Autodesk Inventor part; units mm, degrees
ref_plane "Work Plane1" through (16.75, 3.375, -6.9) normal (1, 0, 0) x (0, 1, 0)
ref_plane "YZ Plane" through (0, 0, 0) normal (1, 0, 0) x (0, 1, 0)
ref_plane "XZ Plane" through (0, 0, 0) normal (0, 1, 0) x (-1, 0, 0)
sketch "Sketch1" plane through (0, 0, 0) normal (0, 1, 0) x (-1, 0, 0)
  line L0 (11.5, 34.5) -> (-11.5, 34.5)
  line L1 (-11.5, 34.5) -> (-11.5, -34.5)
  line L2 (-11.5, -34.5) -> (11.5, -34.5)
  line L3 (11.5, -34.5) -> (11.5, 34.5)
  line L4 (11.5, 34.5) -> (-11.5, -34.5) construction
  line L5 (-11.5, 34.5) -> (11.5, -34.5) construction
  point P0 (0, 0)
  dimension "d0" = 23
  dimension "d1" = 69
extrude "Extrusion1" add sketch "Sketch1" along normal blind 16
sketch "Sketch3" plane through (11.5, 0, 34.5) normal (1, 0, 0) x (0, 0, -1)
  line L0 (0, 0) -> (69, 0)
  line L1 (69, 0) -> (69, 16)
  line L2 (0, 16) -> (69, 16)
  line L3 (0, 0) -> (0, 16)
  line L4 (41.4, 13.119) -> (36.4, 13.119)
  line L5 (36.4, 13.119) -> (36.4, 11.6808)
  line L6 (36.4, 11.6668) -> (36.4, 3.375)
  line L7 (41.4, 2.875) -> (36.4, 2.875)
  line L8 (36.4, 3.375) -> (36.4, 2.875)
  line L9 (0, 0) -> (0, 16)
  line L10 (36.4, 13.119) -> (0, 13.119)
  line L11 (0, 13.119) -> (0, 2.875)
  line L12 (0, 2.875) -> (36.4, 2.875)
  line L13 (36.4, 2.875) -> (36.4, 13.119)
  point P0 (34.5, 0)
ref_plane "Work Plane1" through (16.75, 3.375, -6.9) normal (1, 0, 0) x (0, 1, 0)
extrude "Extrusion2" add sketch "Sketch3" along normal up to surface (5.25 mm away) contours L3 L10 L5 L13 L6 L8 L12
properties part number "bigLipo"
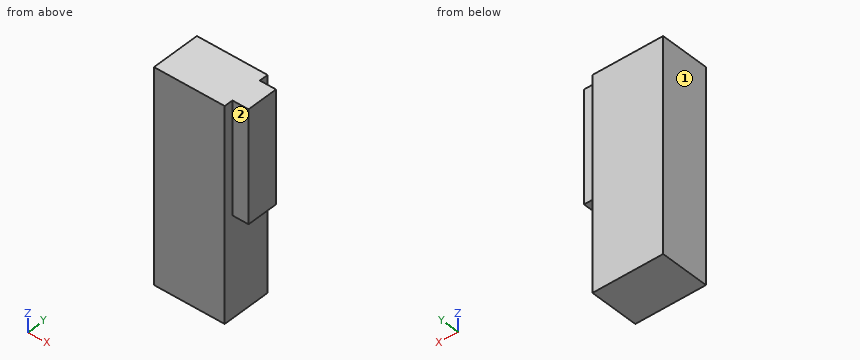
Part model, mm, in its own coordinate system. Face numbers are marked on the shaded views. A direction names the side the tool comes from. Round coordinates to 2 decimals unless told otherwise and drop trailing zeros. Order: outer loops, then holes, each group sorted by start corner. A loop starts at its lowest first (then second) coordinate and runs counter-clockwise, first axis right, second up. Notation, with made-up numbers: M 33,12.5 L 90,12.5 A13 cw 90,31.5 Z; hole C -27.5,70.5 d3. An arc over 180 degrees is marked long. Answer in a Markdown table with one row per item. Add a question column.
Q1. Wall check: L1, parallel to X at y = 10.5, z = -25. Give the ranges that are in metal, low to high. Write a range as from..to.
Q2. Cut at B-B on z = 25.5. Give the cut face in (x, y) (3 decimals), and give its area (3 significant figures).
Q3. Cut at A-A on y = 3.75. Give the cut face in (x, z), and give its area (3 significant figures).
Q4. 3-axis set-ups, long thin cutter, end or side, ignore diameter. For the marked faces 1 and 2: which of +Z, -Z, +X, -X, +Y, -Y reach the whole face in a straight line?
Q5. Cut at D-D on z = -25. Give the cut face in (x, y).
Q6. Cut at C-C on x = 13.5. Give the cut face in (y, z) (3 decimals).
Q7. Pin check, flat tips, straight feed: pin 1 (10 mm diameter, centred on x = 12, z = -15, fed in from +Y); pin 2 (1.6 mm diameter, centred on x = 14.5, z = 17, fed in from +Y). Stop position of each tip, or through.
Established:
| question | item | result |
|---|---|---|
| 1 | L1 | x = -11.5..11.5 |
| 2 | outline | M -11.5,0 L 11.5,0 L 11.5,2.875 L 16.75,2.875 L 16.75,13.119 L 11.5,13.119 L 11.5,16 L -11.5,16 Z |
| 2 | area | 422 mm2 |
| 3 | outline | M -11.5,-34.5 L 11.5,-34.5 L 11.5,-1.9 L 16.75,-1.9 L 16.75,34.5 L -11.5,34.5 Z |
| 3 | area | 1,780 mm2 |
| 4 | face 1 | +Z, -Z, -X, +Y, -Y |
| 4 | face 2 | +Z, -Z, +X, -Y |
| 5 | outline | M -11.5,0 L 11.5,0 L 11.5,16 L -11.5,16 Z |
| 6 | outline | M 2.875,-1.9 L 13.119,-1.9 L 13.119,34.5 L 2.875,34.5 Z |
| 7 | pin 1 | stops at y = 16 |
| 7 | pin 2 | stops at y = 13.12 |
